from build123d import *

# Parameters (mm, degrees)
SKETCH1_W            = 180
SKETCH1_H            = 24
BOSS_EXTRUDE3_DEPTH  = 10
SKETCH1_6_R          = 20
SKETCH1_6_R_2        = 10
HEAD_WIDTH_DEPTH     = 18.75
SKETCH1_7_R          = 20
SKETCH1_7_R_2        = 10
CUT_EXTRUDE1_DEPTH   = 6.25
FILLET1_START        = -6.25
FILLET1_DEPTH        = 12.5
FILLET2_R            = 3.25
SKETCH2_W            = 163.5
SKETCH2_H            = 14
CUT_EXTRUDE2_DEPTH   = 5
FILLET3_R            = 5
FILLET3_OF_MIRROR1_R = 5


with BuildPart() as part:
    # Sketch1 → Boss-Extrude3 (new, symmetric)
    with BuildSketch(Plane.XY):
        with Locations((125, 0)):
            Rectangle(SKETCH1_W, SKETCH1_H)
    extrude(amount=BOSS_EXTRUDE3_DEPTH, both=True)

    # Sketch1<6> → Head Width (add, symmetric)
    # profile 1 of 4: a face of its own
    with BuildSketch(Plane.XY):
        with BuildLine():
            Line((35, -12), (35, 12))
            Line((35, 12), (35, 20))
            Line((35, 20), (0, 20))
            ThreePointArc((0, 20), (14.142135624, 14.142135624), (20, 0))
            ThreePointArc((20, 0), (14.142135624, -14.142135624), (0, -20))
            Line((0, -20), (35, -20))
            Line((35, -20), (35, -12))
        make_face()
    # profile 2 of 4: a face of its own
    with BuildSketch(Plane.XY):
        Circle(SKETCH1_6_R)
        Circle(SKETCH1_6_R_2, mode=Mode.SUBTRACT)
    # profile 3 of 4: a face of its own
    with BuildSketch(Plane.XY):
        with BuildLine():
            Line((215, 20), (215, 12))
            Line((215, 12), (215, -12))
            Line((215, -12), (215, -20))
            Line((215, -20), (250, -20))
            ThreePointArc((250, -20), (230, 0), (250, 20))
            Line((250, 20), (215, 20))
        make_face()
    # profile 4 of 4: a face of its own
    with BuildSketch(Plane.XY):
        with Locations((250, 0)):
            Circle(SKETCH1_6_R)
        with Locations((250, 0)):
            Circle(SKETCH1_6_R_2, mode=Mode.SUBTRACT)
    extrude(amount=HEAD_WIDTH_DEPTH, both=True)

    # Sketch1<7> → Cut-Extrude1 (cut, symmetric)
    # profile 1 of 2: a face of its own
    with BuildSketch(Plane.XY):
        Circle(SKETCH1_7_R)
        Circle(SKETCH1_7_R_2, mode=Mode.SUBTRACT)
    # profile 2 of 2: a face of its own
    with BuildSketch(Plane.XY):
        with Locations((250, 0)):
            Circle(SKETCH1_7_R)
        with Locations((250, 0)):
            Circle(SKETCH1_7_R_2, mode=Mode.SUBTRACT)
    extrude(amount=CUT_EXTRUDE1_DEPTH, both=True, mode=Mode.SUBTRACT)

    # Fillet1: read off the stored shape, not the designer's step
    # Fillet1 outline → Fillet1 (cut)
    with BuildSketch(Plane.XY.offset(FILLET1_START)):
        with BuildLine():
            ThreePointArc((230, 20), (234.472135955, 17.236067977), (234, 12))
            ThreePointArc((234, 12), (241.05572809, 17.88854382), (250, 20))
            Line((250, 20), (230, 20))
        make_face()
        with BuildLine():
            ThreePointArc((234, -12), (234.472135955, -17.236067977), (230, -20))
            Line((230, -20), (250, -20))
            ThreePointArc((250, -20), (241.05572809, -17.88854382), (234, -12))
        make_face()
        with BuildLine():
            ThreePointArc((20, -20), (15.527864045, -17.236067977), (16, -12))
            ThreePointArc((16, -12), (8.94427191, -17.88854382), (0, -20))
            Line((0, -20), (20, -20))
        make_face()
        with BuildLine():
            ThreePointArc((0, 20), (8.94427191, 17.88854382), (16, 12))
            ThreePointArc((16, 12), (15.527864045, 17.236067977), (20, 20))
            Line((20, 20), (0, 20))
        make_face()
    extrude(amount=FILLET1_DEPTH, mode=Mode.SUBTRACT)

    # Fillet2
    fillet2_edges = [part.edges().sort_by_distance(p)[0] for p in [
        (35, 0, 10),
        (35, 20, 0),
        (35, 0, 18.75),
        (35, -20, 0),
        (35, 0, -18.75),
        (215, -20, 0),
        (215, 0, -18.75),
        (215, 20, 0),
        (215, 0, 18.75),
        (215, 0, 10),
        (35, 0, -10),
        (215, 0, -10),
        (215, -12, 0),
        (35, -12, 0),
        (35, 12, 0),
        (215, 12, 0),
    ]]
    fillet(fillet2_edges, radius=FILLET2_R)

    # Sketch2 → Cut-Extrude2 (cut)
    with BuildSketch(Plane.XY.offset(10)):
        with Locations((125, 0)):
            Rectangle(SKETCH2_W, SKETCH2_H)
    cut_extrude2 = extrude(amount=-CUT_EXTRUDE2_DEPTH, mode=Mode.SUBTRACT)

    # Fillet3
    fillet3_edges = [part.edges().sort_by_distance(p)[0] for p in [
        (43.25, -7, 7.5),
        (43.25, 7, 7.5),
        (206.75, 7, 7.5),
        (206.75, -7, 7.5),
    ]]
    fillet(fillet3_edges, radius=FILLET3_R)

    # Mirror1: Cut-Extrude2 across plane
    add(cut_extrude2.mirror(Plane.XY), mode=Mode.SUBTRACT)

    # Fillet3 of Mirror1
    fillet3_of_mirror1_edges = [part.edges().sort_by_distance(p)[0] for p in [
        (43.25, -7, -7.5),
        (43.25, 7, -7.5),
        (206.75, 7, -7.5),
        (206.75, -7, -7.5),
    ]]
    fillet(fillet3_of_mirror1_edges, radius=FILLET3_OF_MIRROR1_R)


solid = part.part
Model file for the job. Use its own axes, mm. A direction names the side the tool comes from. Give positions to 0.01 mm unless a question says otherwise; leave off trailing zeros. Order: outer loops, then holes, each group sorted by start corner. A loop starts at its lowest first (then second) coordinate and runs counter-clockwise, first axis right, second up. Notation, with made-up numbers: (64.5, -13) - (98.5, -13) arc R12 cw to (98.5, -1) - close; hole circle Ø6 at (41, 46). An arc over 180 degrees is marked (long way). Write item = value, one per line. Start each with the question number.
1. Cut at A-A, the plane x = 52. List the corners of the cut face in (y, z).
2. Probe line 1 along Y through (x, z) = (250, -11); line 2 along Y through (x, z) = (125, 9); line 3 along Z through (x, y) = (240, -4). List the from-to ranges inside material, lowest first.
3. Drop flat-ended pins along their axis: P1, Ø9.5, axis at y = 8, z = 2, coming from the -X side; P2, Ø2.5, axis at x = 153, z = 7, coming from the +Y side; P3, Ø2, axis at y = 0, z = 6.5, coming from the +X side. Give the stop position or say it passes through.
4. Two-plate mould, pull along Y, no slides. Class faces 5 (the flat face through (35, -1, 14)), 6 (the cylindrical face through (270, 0, 13)), 7 (the cylindrical face through (230, 0, 0)), 8 (the cylindrical face through (205.32, 5.5, 7.46)): pulls with the +Y half, pulls with the -Y half, needs draft (parallel to the pull), parting line crosses it, or undercut.
5. Which spindle directions (+Z, -Z, +X, -X, +Y, -Y) get a long thin tool onto all of the face, cutting with end or side? Do faces 1 (the flat face through (124, -7, 8)), 2 (the cylindrical face through (234.506, -17.166, -0.088)), 3 (the flat face through (124, 8, -10)), 4 (the cylindrical face through (20, 0, 0)). Say none if no direction does.
Taken from the geometry:
q1.outline = (-12, -10) - (-7, -10) - (-7, -5) - (7, -5) - (7, -10) - (12, -10) - (12, 10) - (7, 10) - (7, 5) - (-7, 5) - (-7, 10) - (-12, 10) - close
q2.line_1 = -20 to -10, 10 to 20
q2.line_2 = -12 to -7, 7 to 12
q2.line_3 = -18.75 to -6.25, 6.25 to 18.75
q3.P1 = -19.12
q3.P2 = 12
q3.P3 = 270
q4.face_5 = needs draft
q4.face_6 = parting line crosses it
q4.face_7 = undercut
q4.face_8 = undercut
q5.face_1 = +Z
q5.face_2 = +X
q5.face_3 = -Z, +Y, -Y
q5.face_4 = -X
